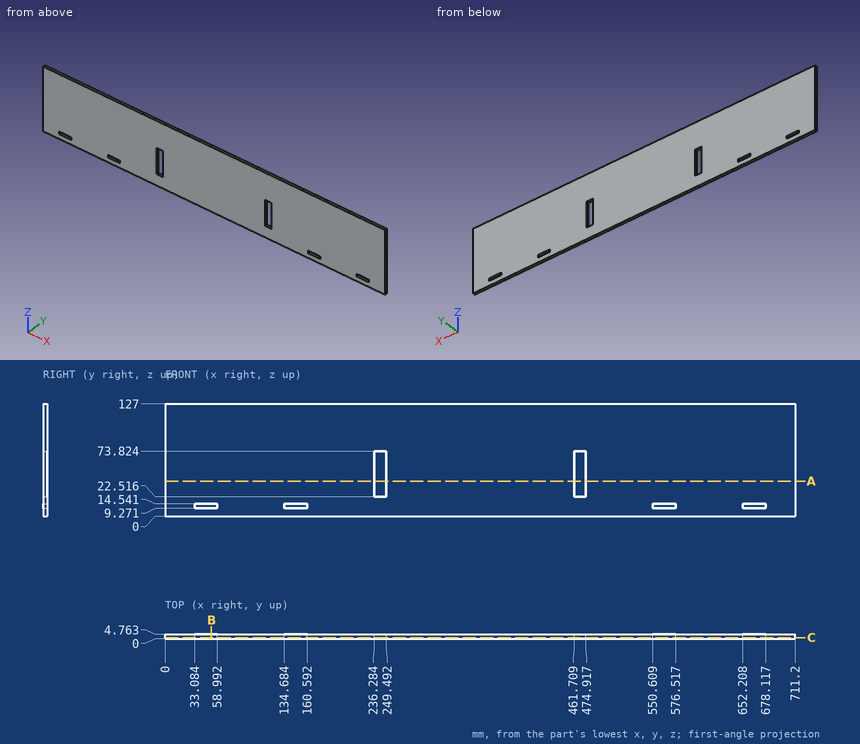
For this review, use the dimensioned drawing (mm, ordinates from the lowest corner) and the shaded views. Give positions to 0.01 mm unless a question says otherwise; leave off trailing zeros. Order: outer loops, then holes, each group sorted by start corner. A loop starts at its lowest first (then second) coordinate and runs counter-clockwise, first axis right, second up.
1. Add section B-B, the plane x = 52. State the section outline as (y, z) points.
Solution:
outline: (0, 0) - (4.76, 0) - (4.76, 9.27) - (0, 9.27) - close; (0, 14.54) - (4.76, 14.54) - (4.76, 127) - (0, 127) - close
2. To check wall thickness, follow L1, parallel to X at y = 1.95, z = 68.5; L2, parallel to X at y = 3.75, z = 12.5; L3, parallel to Z at x = 49, y = 1.9. State the ranges of each line that lie inside material, in increasing order.
Solution:
L1: x = 0 to 236.28, 249.49 to 461.71, 474.92 to 711.2
L2: x = 0 to 33.08, 58.99 to 134.68, 160.59 to 550.61, 576.52 to 652.21, 678.12 to 711.2
L3: z = 0 to 9.27, 14.54 to 127
3. Add section A-A, the plane z = 40. State the section outline as (x, y) points.
Solution:
outline: (0, 0) - (236.28, 0) - (236.28, 4.76) - (0, 4.76) - close; (249.49, 0) - (461.71, 0) - (461.71, 4.76) - (249.49, 4.76) - close; (474.92, 0) - (711.2, 0) - (711.2, 4.76) - (474.92, 4.76) - close
4. Add section C-C, the plane y = 1.2. State the section outline as (x, z) points (1 decimal).
Solution:
outline: (0, 0) - (711.2, 0) - (711.2, 127) - (0, 127) - close; hole (33.1, 9.3) - (59, 9.3) - (59, 14.5) - (33.1, 14.5) - close; hole (134.7, 9.3) - (160.6, 9.3) - (160.6, 14.5) - (134.7, 14.5) - close; hole (236.3, 22.5) - (249.5, 22.5) - (249.5, 73.8) - (236.3, 73.8) - close; hole (461.7, 22.5) - (474.9, 22.5) - (474.9, 73.8) - (461.7, 73.8) - close; hole (550.6, 9.3) - (576.5, 9.3) - (576.5, 14.5) - (550.6, 14.5) - close; hole (652.2, 9.3) - (678.1, 9.3) - (678.1, 14.5) - (652.2, 14.5) - close
